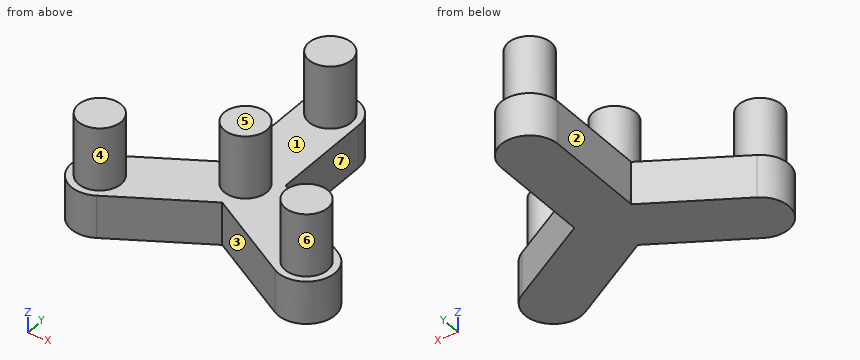
from build123d import *

# Parameters (mm, degrees)
CARRIER_BASE_DEPTH  = 7.5
SKETCH3_R           = 7.5
PLANET_SHAFTS_DEPTH = 22
SKETCH4_R           = 7.5
SUN_SHAFT_DEPTH     = 22


with BuildPart() as part:
    # Sketch1 → Carrier Base (new, symmetric)
    with BuildSketch(Plane.XY):
        with BuildLine():
            Line((0, -11.547005384), (-31.373066961, -29.660254039))
            ThreePointArc((-31.373066961, -29.660254039), (-45.033320997, -26), (-41.373066961, -12.339745963))
            Line((-41.373066961, -12.339745963), (-10, 5.773502692))
            Line((-10, 5.773502692), (-10, 42.000000002))
            ThreePointArc((-10, 42.000000002), (0, 52), (10, 42.000000002))
            Line((10, 42.000000002), (10, 5.773502692))
            Line((10, 5.773502692), (41.373066961, -12.339745963))
            ThreePointArc((41.373066961, -12.339745963), (45.033320997, -26), (31.373066961, -29.660254039))
            Line((31.373066961, -29.660254039), (0, -11.547005384))
        make_face()
    extrude(amount=CARRIER_BASE_DEPTH, both=True)

    # Sketch3 → Planet Shafts (add)
    with BuildSketch(Plane.XY.offset(7.5)):
        with Locations((0, 42)):
            Circle(SKETCH3_R)
        with Locations((36.373066959, -21)):
            Circle(SKETCH3_R)
        with Locations((-36.373066959, -21)):
            Circle(SKETCH3_R)
    extrude(amount=PLANET_SHAFTS_DEPTH)

    # Sketch4 → Sun Shaft (add)
    with BuildSketch(Plane.XY.offset(7.5)):
        Circle(SKETCH4_R)
    extrude(amount=SUN_SHAFT_DEPTH)


solid = part.part
Verification items for the finished model (mm, model axes). Face numbers are marked on the shaded views. A direction names the side the tool comes from. Give positions to 0.01 mm unless a question says otherwise; leave off trailing zeros. Order: outer loops, then holes, each group sorted by start corner. A loop starts at its lowest first (then second) coordinate and runs counter-clockwise, first axis right, second up. Notation, with made-up numbers: M 54,44 L 102,44 A7 ccw 102,48 Z; hole C 72,33 d7. An arc over 180 degrees is marked long. Answer as a JSON object with one key per item and string values. Group by question number.
1) Cross-section at C-C (z = 13.5). Enter the section's corners in (x, y).
2) Cross-section at B-B (z = 4). Enter the section's corners in (x, y).
3) Scan lines: line 1 along Y through (x, z) = (0.5, 27); line 2 along X through (y, z) = (0.5, 8.5); line 3 along X through (y, z) = (13, 2.5). Record each from-to range of solid material in increasing order. Write a range as [from, to].
4) Mould release check, pull along X, two halves, no side actions. Record for the marked faces 4, 5, 6 and 7: released by +X, released by -X, zero draft, split by the parting line, or undercut.
5) Access from +Z, -Z, +X, -X, +Y, -Y to the whole of each face (thin tool, end or side, straight path). Record for the marked faces 1, 2 and 3.
6) Depth check by flat-ended pin: pin 1 Ø3 at (y, z) = (-8, 22) entering from +X; pin 2 Ø6 at (x, z) = (-8.5, 7) entering from -Y; pin 3 Ø12 at (x, z) = (26, 3.5) entering from +Y. Enter the tip coordinate at first touch or a pass-through.
7) Cross-section at D-D (x = -39). Enter the section's corners in (y, z).
8) Cross-section at A-A (y = 0). Enter the section's corners in (x, z).
Result sheet:
{
 "1": {"outline": "C -36.37,-21 d15; C 0,0 d15; C 0,42 d15; C 36.37,-21 d15"},
 "2": {"outline": "M -41.37,-12.34 A10 ccw -31.37,-29.66 L 0,-11.55 L 31.37,-29.66 A10 ccw 41.37,-12.34 L 10,5.77 L 10,42 A10 ccw -10,42 L -10,5.77 Z"},
 "3": {"line 1": "y = [-7.48, 7.48], [34.52, 49.48]", "line 2": "x = [-7.48, 7.48]", "line 3": "x = [-10, 10]"},
 "4": {"face 4": "undercut", "face 5": "zero draft", "face 6": "undercut", "face 7": "released by +X"},
 "5": {"face 1": "+Z", "face 2": "+Z, -Z, -X, +Y", "face 3": "+Z, -Z, -Y"},
 "6": {"pin 1": "stops at x = 3.74", "pin 2": "stops at y = -18.19", "pin 3": "stops at y = 0"},
 "7": {"outline": "M -30.65,-7.5 L -10.97,-7.5 L -10.97,7.5 L -13.98,7.5 L -13.98,29.5 L -28.02,29.5 L -28.02,7.5 L -30.65,7.5 Z"},
 "8": {"outline": "M -20,-7.5 L 20,-7.5 L 20,7.5 L 7.5,7.5 L 7.5,29.5 L -7.5,29.5 L -7.5,7.5 L -20,7.5 Z"}
}
